The model under review builds one solid part; all positions refer to its coordinate system, in mm. A direction names the side the tool comes from. Coordinates: 2 decimals unless noted, no trailing zeros. Write each loop counter-clockwise with the first axis right and the second up, starting at its lowest first coordinate (ties: lowest second). Pieces come first, ordered by that corner, then holes. Notation, with made-up numbers: M -27.5,44 L -7.5,44 A18 cw -7.5,50 Z; hole C 47.5,-17.5 d2. An arc over 180 degrees is marked long. Answer as CSV lines item,"result". Start each with the question number.
from build123d import *

# Parameters (mm, degrees)
SKETCH1_R           = 19.75
SKETCH1_R_2         = 1.25
BOSS_EXTRUDE1_DEPTH = 3
BOSS_EXTRUDE2_START = 22
SKETCH2_R           = 2
BOSS_EXTRUDE2_DEPTH = 22
SKETCH5_R           = 8
CUT_EXTRUDE1_DEPTH  = 3
SKETCH6_R           = 9
CUT_EXTRUDE2_DEPTH  = 2
FILLET2_R           = 2
SKETCH10_R          = 2.7
CUT_EXTRUDE4_DEPTH  = 4
CHAMFER1_SIZE       = 0.5
CUT_EXTRUDE5_DEPTH  = 22
SKETCH14_R          = 5.5
SKETCH14_R_2        = 7
CUT_EXTRUDE6_DEPTH  = 87.788536135


with BuildPart() as part:
    # Sketch1 → Boss-Extrude1 (new body)
    with BuildSketch(Plane.XY):
        with BuildLine():
            Line((-66.5, 44), (66.5, 44))
            ThreePointArc((66.5, 44), (70.035533906, 42.535533906), (71.5, 39))
            Line((71.5, 39), (71.5, -39))
            ThreePointArc((71.5, -39), (70.035533906, -42.535533906), (66.5, -44))
            Line((66.5, -44), (-66.5, -44))
            ThreePointArc((-66.5, -44), (-70.035533906, -42.535533906), (-71.5, -39))
            Line((-71.5, -39), (-71.5, 39))
            ThreePointArc((-71.5, 39), (-70.035533906, 42.535533906), (-66.5, 44))
        make_face()
        with Locations((43.5, 16)):
            Circle(SKETCH1_R, mode=Mode.SUBTRACT)
        with Locations((27.25, 32.25)):
            Circle(SKETCH1_R_2, mode=Mode.SUBTRACT)
        with Locations((59.75, 32.25)):
            Circle(SKETCH1_R_2, mode=Mode.SUBTRACT)
        with Locations((59.75, -0.25)):
            Circle(SKETCH1_R_2, mode=Mode.SUBTRACT)
        with Locations((27.25, -0.25)):
            Circle(SKETCH1_R_2, mode=Mode.SUBTRACT)
    extrude(amount=BOSS_EXTRUDE1_DEPTH)

    # Sketch2 → Boss-Extrude2 (add)
    with BuildSketch(Plane(origin=(0, 0, 0), x_dir=(-1, 0, 0), z_dir=(0, 0, -1)).offset(BOSS_EXTRUDE2_START)):
        with BuildLine():
            Line((-66.5, 44), (66.5, 44))
            ThreePointArc((66.5, 44), (70.035533906, 42.535533906), (71.5, 39))
            Line((71.5, 39), (71.5, -39))
            ThreePointArc((71.5, -39), (70.035533906, -42.535533906), (66.5, -44))
            Line((66.5, -44), (-66.5, -44))
            ThreePointArc((-66.5, -44), (-70.035533906, -42.535533906), (-71.5, -39))
            Line((-71.5, -39), (-71.5, 39))
            ThreePointArc((-71.5, 39), (-70.035533906, 42.535533906), (-66.5, 44))
        make_face()
        with Locations((-66.5, 39)):
            Circle(SKETCH2_R, mode=Mode.SUBTRACT)
        with Locations(Location((66.5, 39, 0), (0, 0, 180))):
            Circle(SKETCH2_R, mode=Mode.SUBTRACT)
        with Locations((66.5, -39)):
            Circle(SKETCH2_R, mode=Mode.SUBTRACT)
        with Locations(Location((-66.5, -39, 0), (0, 0, 180))):
            Circle(SKETCH2_R, mode=Mode.SUBTRACT)
        with BuildLine():
            Line((-61.917424305, 41), (61.917424305, 41))
            Line((61.917424305, 41), (61.917424305, 37))
            ThreePointArc((61.917424305, 37), (64.673843213, 34.345416088), (68.5, 34.417424305))
            Line((68.5, 34.417424305), (68.5, -34.417424305))
            ThreePointArc((68.5, -34.417424305), (64.673843213, -34.345416088), (61.917424305, -37))
            Line((61.917424305, -37), (61.917424305, -41))
            Line((61.917424305, -41), (-61.917424305, -41))
            ThreePointArc((-61.917424305, -41), (-62.964466094, -35.464466094), (-68.5, -34.417424305))
            Line((-68.5, -34.417424305), (-68.5, 34.417424305))
            ThreePointArc((-68.5, 34.417424305), (-62.964466094, 35.464466094), (-61.917424305, 41))
        make_face(mode=Mode.SUBTRACT)
    extrude(amount=-BOSS_EXTRUDE2_DEPTH)

    # Sketch5 → Cut-Extrude1 (cut)
    with BuildSketch(Plane(origin=(71.5, 0, 0), x_dir=(0, 0, -1), z_dir=(1, 0, 0))):
        with Locations(Location((11, -23, 0), (0, 0, 90))):
            Circle(SKETCH5_R)
    extrude(amount=-CUT_EXTRUDE1_DEPTH, mode=Mode.SUBTRACT)

    # Sketch6 → Cut-Extrude2 (cut)
    with BuildSketch(Plane(origin=(71.5, 0, 0), x_dir=(0, 0, -1), z_dir=(1, 0, 0))):
        with Locations(Location((11, -23, 0), (0, 0, 90))):
            Circle(SKETCH6_R)
    extrude(amount=-CUT_EXTRUDE2_DEPTH, mode=Mode.SUBTRACT)

    # Fillet2
    fillet2_edges = [part.edges().sort_by_distance(p)[0] for p in [
        (-70.035533906, -42.535533906, 3),
        (0, -44, 3),
        (70.035533906, -42.535533906, 3),
        (71.5, 0, 3),
        (70.035533906, 42.535533906, 3),
        (0, 44, 3),
        (-70.035533906, 42.535533906, 3),
        (0, 41, 0),
        (68.5, 0, 0),
        (0, -41, 0),
        (-68.5, 0, 0),
        (-71.5, 0, 3),
    ]]
    fillet(fillet2_edges, radius=FILLET2_R)

    # Sketch10 → Cut-Extrude4 (cut)
    with BuildSketch(Plane(origin=(0, 0, -22), x_dir=(-1, 0, 0), z_dir=(0, 0, -1))):
        with Locations((-66.5, 39)):
            Circle(SKETCH10_R)
        with Locations((66.5, 39)):
            Circle(SKETCH10_R)
        with Locations((66.5, -39)):
            Circle(SKETCH10_R)
        with Locations((-66.5, -39)):
            Circle(SKETCH10_R)
    extrude(amount=-CUT_EXTRUDE4_DEPTH, mode=Mode.SUBTRACT)

    # Chamfer1
    chamfer1_edges = [part.edges().sort_by_distance(p)[0] for p in [
        (69.2, -39, -22),
        (-63.8, -39, -22),
        (-63.8, 39, -22),
        (69.2, 39, -22),
    ]]
    chamfer(chamfer1_edges, length=CHAMFER1_SIZE)

    # Sketch11 → Cut-Extrude5 (cut)
    with BuildSketch(Plane(origin=(0, 0, -22), x_dir=(-1, 0, 0), z_dir=(0, 0, -1))):
        with BuildLine():
            Line((-63.75, 34.75), (-62.25, 34.75))
            Line((-62.25, 34.75), (-62.25, 36.25))
            ThreePointArc((-62.25, 36.25), (-63.310660172, 35.810660172), (-63.75, 34.75))
        make_face()
    extrude(amount=-CUT_EXTRUDE5_DEPTH, mode=Mode.SUBTRACT)

    # Sketch14 → Cut-Extrude6 (cut, through all)
    with BuildSketch(Plane(origin=(0, 0, 0), x_dir=(-1, 0, 0), z_dir=(0, 0, -1))):
        with Locations((41.5, 24)):
            Circle(SKETCH14_R)
        with Locations((11.5, 24)):
            Circle(SKETCH14_R_2)
    extrude(amount=-CUT_EXTRUDE6_DEPTH, mode=Mode.SUBTRACT)


solid = part.part
1) Tool access review of faces 4 (the flat face through (67, 39, 0)), 5 (the cylindrical face through (69.007, -29.349, -15.868)), 6 (the cylindrical face through (70, -42.57, -10.66)): name each direction out of +Z, -Z, +X, -X, +Y, -Y from which nothing blocks a thin tool from reaching the whole face with its end or side.
2) Take a section at D-D on x = -34. Give the boundary of the cut face in (y, z).
3) Take a section at A-A on x = -11.5. Give the boundary of the cut face in (y, z).
4) Clearance check with flat-ended pins moving along their axes: pin 1 Ø10 at (x, y) = (-41.5, 24) entering from +Z; pin 2 Ø6 at (x, y) = (68, -38) entering from -Z; pin 3 Ø6 at (x, y) = (-66.5, 39) entering from -Z; pin 4 Ø1.6 at (x, y) = (-67.5, -37.5) entering from -Z. State where each tip first meets the part, or that it passes through.
5) Mouldability with a two-part tool opening along Z and no side actions: class faces 1 (the flat face through (-64, 39, -18)), 2 (the cylindrical face through (70.514, -14.686, -14.447)), 3 (the cylindrical face through (67.085, -41.636, -19.774)) as +Z half, -Z half, draft (parallel to the pull), parting line (faces both ways), or undercut.
6) Take a section at C-C on z = -13. Give the number of separate pieces and of enclosed holes in the cut face, and give its area (3 significant figures).
7) Take a section at B-B on y = -23. Give the boundary of the cut face in (x, z).
8) To check wall thickness, follow line 1 (Y direction, x = 66.5, z = -11.75); line 2 (Y direction, x = -58, z = -8); line 3 (Y direction, x = -41.5, z = 1.05). State the ranges of each line that lie inside material, in increasing order. Write a range as [from, to].
Results:
1,face 4,"-Z"
1,face 5,"+X"
1,face 6,"+Z, -Z, +X, -Y"
2,outline,"M -44,-22 L -41,-22 L -41,-2 A2 cw -39,0 L 39,0 A2 cw 41,-2 L 41,-22 L 44,-22 L 44,1 A2 ccw 42,3 L -42,3 A2 ccw -44,1 Z"
3,outline,"M -44,-22 L -41,-22 L -41,-2 A2 cw -39,0 L 17,0 L 17,3 L -42,3 A2 ccw -44,1 Z; M 31,0 L 39,0 A2 cw 41,-2 L 41,-22 L 44,-22 L 44,1 A2 ccw 42,3 L 31,3 Z"
4,pin 1,"passes through"
4,pin 2,"stops at z = -22"
4,pin 3,"stops at z = -21.8"
4,pin 4,"stops at z = -18"
5,face 1,"-Z half"
5,face 2,"undercut"
5,face 3,"draft"
6,separate pieces,"1"
6,enclosed holes,"4"
6,area,"1,400 mm²"
7,outline,"M -71.5,-22 L -68.5,-22 L -68.5,-2 A2 cw -66.5,0 L 66.5,0 A2 cw 68.5,-2 L 68.5,-3 L 69.5,-3 L 69.5,-2 L 71.5,-2 L 71.5,1 A2 ccw 69.5,3 L -69.5,3 A2 ccw -71.5,1 Z; M 68.5,-22 L 71.5,-22 L 71.5,-20 L 69.5,-20 L 69.5,-19 L 68.5,-19 Z"
8,line 1,"y = [-44, -41], [-37, -34], [34, 37], [41, 44]"
8,line 2,"y = [-44, -41], [41, 44]"
8,line 3,"y = [-44, 18.5], [29.5, 44]"
